from build123d import *

# Parameters (mm, degrees)
SKETCH_1_R          = 1.35
SKETCH_1_R_2        = 1.6
SKETCH_1_W          = 10.785023523
SKETCH_1_H          = 3.975869969
SKETCH_1_W_2        = 3.881137471
SKETCH_1_H_2        = 6.926362959
SKETCH_1_H_3        = 6.753909589
SKETCH_1_W_3        = 2.381
SKETCH_1_H_4        = 1.694
SKETCH_1_W_4        = 2.327
SKETCH_1_H_5        = 1.693
SKETCH_1_W_5        = 24.737091535
SKETCH_1_H_6        = 13.600314953
SKETCH_1_W_6        = 15.83465493
SKETCH_1_W_7        = 3.735479659
EXTRUDE_1_DEPTH     = 3
SKETCH_2_R          = 1.6
CUT_EXTRUDE_1_DEPTH = 55.763647529


with BuildPart() as part:
    # 草图1 → 凸台-拉伸1 (new body)
    with BuildSketch(Plane(origin=(0, 0, 0), x_dir=(-1, 0, 0), z_dir=(0, 0, -1))):
        with BuildLine():
            Line((28.933183464, 3), (28.933183464, 41.999))
            ThreePointArc((28.933183464, 41.999), (28.054503808, 44.120320344), (25.933183464, 44.999))
            Line((25.933183464, 44.999), (-28.066816536, 44.999))
            ThreePointArc((-28.066816536, 44.999), (-30.18813688, 44.120320344), (-31.066816536, 41.999))
            Line((-31.066816536, 41.999), (-31.066816536, 3))
            ThreePointArc((-31.066816536, 3), (-30.18813688, 0.878679656), (-28.066816536, 0))
            Line((-28.066816536, 0), (25.933183464, 0))
            ThreePointArc((25.933183464, 0), (28.054503808, 0.878679656), (28.933183464, 3))
        make_face()
        with Locations(Location((-26.567767322, 12.499, 0), (0, 0, 180))):
            Circle(SKETCH_1_R, mode=Mode.SUBTRACT)
        with Locations(Location((-10.567816536, 23.43, 0), (0, 0, 180))):
            Circle(SKETCH_1_R_2, mode=Mode.SUBTRACT)
        with Locations(Location((24.432183464, 12.499, 0), (0, 0, 180))):
            Circle(SKETCH_1_R, mode=Mode.SUBTRACT)
        with Locations(Location((-10.567816536, 42.43, 0), (0, 0, 180))):
            Circle(SKETCH_1_R_2, mode=Mode.SUBTRACT)
        with Locations((16.376273559, 4.440236649)):
            Rectangle(SKETCH_1_W, SKETCH_1_H, mode=Mode.SUBTRACT)
        with Locations((24.382587874, 5.915483144)):
            Rectangle(SKETCH_1_W_2, SKETCH_1_H_2, mode=Mode.SUBTRACT)
        with Locations((24.382587874, 19.014796064)):
            Rectangle(SKETCH_1_W_2, SKETCH_1_H_3, mode=Mode.SUBTRACT)
        with Locations((18.298683464, 30.257)):
            Rectangle(SKETCH_1_W_3, SKETCH_1_H_4, mode=Mode.SUBTRACT)
        with Locations((18.271683464, 35.4965)):
            Rectangle(SKETCH_1_W_4, SKETCH_1_H_5, mode=Mode.SUBTRACT)
        with Locations((-10.43601502, 32.923896791)):
            Rectangle(SKETCH_1_W_5, SKETCH_1_H_6, mode=Mode.SUBTRACT)
        with Locations((-16.015517123, 4.440236649)):
            Rectangle(SKETCH_1_W_6, SKETCH_1_H, mode=Mode.SUBTRACT)
        with Locations((-26.559738671, 5.915483144)):
            Rectangle(SKETCH_1_W_7, SKETCH_1_H_2, mode=Mode.SUBTRACT)
        with Locations((-26.559738671, 19.014796064)):
            Rectangle(SKETCH_1_W_7, SKETCH_1_H_3, mode=Mode.SUBTRACT)
    extrude(amount=-EXTRUDE_1_DEPTH)

    # 草图2 → 切除-拉伸1 (cut, through all)
    with BuildSketch(Plane.XY.offset(3)):
        with Locations((-24.432183464, 12.499)):
            Circle(SKETCH_2_R)
        with Locations((26.567767322, 12.499)):
            Circle(SKETCH_2_R)
    extrude(amount=-CUT_EXTRUDE_1_DEPTH, mode=Mode.SUBTRACT)


solid = part.part
Source: CAD feature listing. Evaluate the final solid. Frame: model axes, mm. A direction names the side the tool comes from. Coordinates: 2 decimals unless noted, no trailing zeros. Loops run counter-clockwise (first coordinate to the right, second up) from the corner with the lowest first, then second, coordinate; pieces in that order, holes last. Notation, with made-up numbers: (88.25, 74.5) - (124.25, 74.5) arc R10 cw to (124.25, 85.5) - close; hole circle Ø11 at (81.25, 57.5). An arc over 180 degrees is marked (long way). One line per question, with ' | ' between items.
1) Pull-direction query (X, two-part tool) for faces 1 (the face through (31.067, 23, 1)), 2 (the face through (-16, 2.452, 1)), 3 (the face through (1, 44.999, 1)); classes: released by +X, released by -X, zero draft, split by the parting line, or undercut.
Report:
face 1: released by +X | face 2: undercut | face 3: zero draft
2) Section C-C, the plane z = 2.1. Give the number of separate pieces and of enclosed holes in the cut face, then the cut area to 3 significant figures.
Report:
separate pieces: 1 | enclosed holes: 13 | area: 2,110 mm²
3) Line query: line 1 along Y through (x, z) = (12.5, 2.85); line 2 along X through (y, z) = (8, 2.3); line 3 along Y through (x, z) = (-23.5, 2.6). Output: solid intervals per line, ascending.
Report:
line 1: y = 0 to 2.45, 6.43 to 26.12, 39.72 to 45 | line 2: x = -28.93 to -26.32, -22.44 to 24.69, 28.43 to 31.07 | line 3: y = 0 to 2.45, 9.38 to 11.2, 13.8 to 15.64, 22.39 to 45
4) Set-up query: faces 4 (the face through (-22.442, 19, 1)), 5 (the face through (-28.933, 22, 1)). Return all of +Z, -Z, +X, -X, +Y, -Y with unobstructed straight access to the full face (end or side cutting, diameter ignored); none if empty.
Report:
face 4: +Z, -Z | face 5: +Z, -Z, -X, +Y, -Y
5) Section A-A, the plane y = 19.5. Return loops of the section in (x, z), then the cut area to 3 significant figures.
Report:
outline: (-28.93, 0) - (-26.32, 0) - (-26.32, 3) - (-28.93, 3) - close; (-22.44, 0) - (24.69, 0) - (24.69, 3) - (-22.44, 3) - close; (28.43, 0) - (31.07, 0) - (31.07, 3) - (28.43, 3) - close | area: 157 mm²
6) Section B-B, the plane y = 32. Return loops of the section in (x, z), then the cut area to 3 significant figures.
Report:
outline: (-28.93, 0) - (-1.93, 0) - (-1.93, 3) - (-28.93, 3) - close; (22.8, 0) - (31.07, 0) - (31.07, 3) - (22.8, 3) - close | area: 106 mm²
